Model file for the job. Use its own axes, mm. A direction names the side the tool comes from. Give positions to 0.01 mm unless a question says otherwise; leave off trailing zeros. Loops run counter-clockwise (first coordinate to the right, second up) from the corner with the lowest first, then second, coordinate; pieces in that order, holes last. Notation, with made-up numbers: M -5,-23 L 18,-23 A14 ccw 18,0 Z; hole C 13,27 d8. An arc over 180 degrees is marked long. Answer in a Markdown table with one row per item.
```python
from build123d import *

# Parameters (mm, degrees)
SKETCH1_W           = 32
SKETCH1_H           = 16
BOSS_EXTRUDE1_DEPTH = 36
SKETCH2_W           = 32
SKETCH2_H           = 12.8
CUT_EXTRUDE1_DEPTH  = 1.6
SKETCH3_R           = 6.05
CUT_EXTRUDE2_DEPTH  = 44.036739415


with BuildPart() as part:
    # Sketch1 → Boss-Extrude1 (new body)
    with BuildSketch(Plane(origin=(0, 0, 0), x_dir=(1, 0, 0), z_dir=(0, 1, 0))):
        with Locations((1.325153374, -1.104294479)):
            Rectangle(SKETCH1_W, SKETCH1_H)
    extrude(amount=BOSS_EXTRUDE1_DEPTH)

    # Sketch2 → Cut-Extrude1 (cut)
    with BuildSketch(Plane(origin=(0, 0, 0), x_dir=(-1, 0, 0), z_dir=(0, -1, 0))):
        with Locations((-1.325153374, -1.104294479)):
            Rectangle(SKETCH2_W, SKETCH2_H)
    extrude(amount=-CUT_EXTRUDE1_DEPTH, mode=Mode.SUBTRACT)

    # Sketch3 → Cut-Extrude2 (cut, through all)
    with BuildSketch(Plane(origin=(0, 0, -6.895705521), x_dir=(-1, 0, 0), z_dir=(0, 0, -1))):
        with Locations((-1.325153374, 24.5)):
            Circle(SKETCH3_R)
    extrude(amount=-CUT_EXTRUDE2_DEPTH, mode=Mode.SUBTRACT)


solid = part.part
```
(1) Which spindle directions (+Z, -Z, +X, -X, +Y, -Y) get a long thin tool onto all of the face, cutting with end or side? Do faces 1 (the flat face through (1, 0, -6)), 2 (the flat face through (2, 1.6, 1)). Say none if no direction does.
Established:
| item | result |
|---|---|
| face 1 | +Z, -Z, +X, -X, -Y |
| face 2 | +X, -X, -Y |
(2) Saw through at B-B, the plane x = -1. Give the cut face in (y, z), and give its area (3 significant figures).
Established:
| item | result |
|---|---|
| outline | M 0,-6.9 L 18.91,-6.9 L 18.91,9.1 L 0,9.1 L 0,7.5 L 1.6,7.5 L 1.6,-5.3 L 0,-5.3 Z; M 30.09,-6.9 L 36,-6.9 L 36,9.1 L 30.09,9.1 Z |
| area | 377 mm2 |
(3) Flat gauge pins, fed straight in: P1, Ø6, axis at x = 10, z = -1, coming from the -Y side; P2, Ø11, axis at x = 1.33, y = 24.5, coming from the +Z side. Where does each tip first touch, or does it go through?
Established:
| item | result |
|---|---|
| P1 | stops at y = 1.6 |
| P2 | passes through |
(4) Saw through at D-D, the plane y = 30. Give the cut face in (x, z), and give its area (3 significant figures).
Established:
| item | result |
|---|---|
| outline | M -14.67,-6.9 L -1.2,-6.9 L -1.2,9.1 L -14.67,9.1 Z; M 3.85,-6.9 L 17.33,-6.9 L 17.33,9.1 L 3.85,9.1 Z |
| area | 431 mm2 |
(5) Saw through at A-A, the plane y = 24.5. Give the cut face in (x, z).
Established:
| item | result |
|---|---|
| outline | M -14.67,-6.9 L -4.72,-6.9 L -4.72,9.1 L -14.67,9.1 Z; M 7.38,-6.9 L 17.33,-6.9 L 17.33,9.1 L 7.38,9.1 Z |
(6) Saw through at C-C, the plane z = -4.5. Give the cut face in (x, y).
Established:
| item | result |
|---|---|
| outline | M -14.67,1.6 L 17.33,1.6 L 17.33,36 L -14.67,36 Z; hole C 1.33,24.5 d12.1 |
(7) Wall check: L1, parallel to Y at x = 8, z = 1.75; L2, parallel to X at y = 30, z = 7.5; L3, parallel to X at y = 28, z = -1.5. Give the ranges that are in metal, low to high.
Established:
| item | result |
|---|---|
| L1 | y = 1.6 to 36 |
| L2 | x = -14.67 to -1.2, 3.85 to 17.33 |
| L3 | x = -14.67 to -3.61, 6.26 to 17.33 |
(8) Mould opens along Z. For faces 3 (the flat face through (2, 1, 7.504)), 4 (the flat face through (1, 18, -6.896)), 5 (the flat face through (1, 18, 9.104)), 6 (the flat face through (-14.675, 18, 1)) say: pulls with the +Z half, pulls with the -Z half, needs draft (parallel to the pull), parting line crosses it, or undercut.
Established:
| item | result |
|---|---|
| face 3 | undercut |
| face 4 | pulls with the -Z half |
| face 5 | pulls with the +Z half |
| face 6 | needs draft |
